Verification items for the finished model (mm, model axes). Coordinates: 2 decimals unless noted, no trailing zeros. Write each loop counter-clockwise with the first axis right and the second up, starting at its lowest first coordinate (ties: lowest second). Pieces come first, ordered by that corner, then holes. Notation, with made-up numbers: M 79.25,69 L 93.25,69 A21 cw 93.25,77 Z; hole C -30.75,19 d8. An arc over 180 degrees is marked long. Answer in a Markdown table with one row per item.
from build123d import *

# Parameters (mm, degrees)
SKETCH_1_R          = 20
EXTRUDE_1_DEPTH     = 20
SKETCH_4_R          = 2.5
CUT_EXTRUDE_1_DEPTH = 35.641016325
CHAMFER_1_SIZE      = 2
CHAMFER_1_SIZE2     = 1.154700538


with BuildPart() as part:
    # 草图1 → 凸台-拉伸1 (new body)
    with BuildSketch(Plane(origin=(0, 0, 0), x_dir=(1, 0, 0), z_dir=(0, 1, 0))):
        with Locations(Location((0, 0, 0), (0, 0, 270))):
            Circle(SKETCH_1_R)
    extrude(amount=EXTRUDE_1_DEPTH)

    # 草图2 → 切除-旋转1 (revolve, cut)
    with BuildSketch(Plane(origin=(0, 20, 0), x_dir=(1, 0, 0), z_dir=(0, 1, 0))):
        with BuildLine():
            Line((0, -3), (0, -23))
            ThreePointArc((0, -23), (-10, -13), (0, -3))
        make_face()
    revolve(axis=Axis((0, 20, 3), (0, 0, 1)), mode=Mode.SUBTRACT)

    # 草图4 → 切除-拉伸1 (cut, through all)
    with BuildSketch(Plane.XZ):
        with Locations(Location((0, -11.5, 0), (0, 0, 270))):
            Circle(SKETCH_4_R)
        with Locations(Location((11.5, 0, 0), (0, 0, 270))):
            Circle(SKETCH_4_R)
        with Locations(Location((-11.5, 0, 0), (0, 0, 270))):
            Circle(SKETCH_4_R)
    extrude(amount=-CUT_EXTRUDE_1_DEPTH, mode=Mode.SUBTRACT)

    # 倒角1
    chamfer_1_edges = [part.edges().sort_by_distance(p)[0] for p in [
        (0, 0, -9),
        (11.5, 0, 2.5),
        (-11.5, 0, 2.5),
    ]]
    chamfer_1_side = [part.faces().sort_by_distance(p)[0] for p in [
        (0, 0, 0.18852459),
    ]]
    chamfer(chamfer_1_edges, length=CHAMFER_1_SIZE, length2=CHAMFER_1_SIZE2, reference=chamfer_1_side[0])


solid = part.part
1) Thickness scan on L1, parallel to X at y = 13, z = 0; L2, parallel to X at y = 11.25, z = -0.5; L3, parallel to Z at x = 2, y = 11.5. Record the ranges inside material, lowest first. Write a range as [from, to].
Response values:
| item | result |
|---|---|
| L1 | x = [-20, -14], [-9, 9], [14, 20] |
| L2 | x = [-19.99, -13.95], [-9.05, 9.05], [13.95, 19.99] |
| L3 | z = [-19.9, -13], [-10, 8.13], [17.87, 19.9] |
2) Depth check by flat-ended pin: pin 1 (1.5 mm diameter, centred on x = 13.5, z = -2.5, fed in from -Y); pin 2 (3 mm diameter, centred on x = 11, y = 13.5, fed in from +Z); pin 3 (6 mm diameter, centred on y = 7.5, z = -11, fed in from +X); pin 4 (12 mm diameter, centred on x = 5, y = 7.5, fed in from -Z). Enter the tip coordinate at first touch or a pass-through.
Response values:
| item | result |
|---|---|
| pin 1 | stops at y = 0.32 |
| pin 2 | stops at z = 17.6 |
| pin 3 | stops at x = 18.33 |
| pin 4 | stops at z = -20 |
3) Release check for a two-part mould opening along Z. For faces 1 (the face through (0, 10, -9)), 2 (the face through (-13.94, 10.45, 0.54)), 3 (the face through (0, 20, -5)), 4 (the face through (0.88, 9.86, -19.98)) record: +Z half, -Z half, draft (parallel to the pull), parting line (faces both ways), or undercut.
Response values:
| item | result |
|---|---|
| face 1 | undercut |
| face 2 | undercut |
| face 3 | draft |
| face 4 | parting line |
4) Sectioned sample at D-D (y = 15.25). Record the cut outline in (x, z), then the cut area to 3 significant figures.
Response values:
| item | result |
|---|---|
| outline | M -6.52,18.91 A20 ccw long 6.52,18.91 A8.8 cw long Z; hole C -11.5,0 d5; hole C 0,-11.5 d5; hole C 11.5,0 d5 |
| area | 971 mm² |
5) Sectioned sample at B-B (z = 0). Record the cut outline in (x, y), then the cut area to 3 significant figures.
Response values:
| item | result |
|---|---|
| outline | M -20,0 L -16,0 L -14,1.15 L -14,20 L -20,20 Z; M -9,1.15 L -7,0 L 7,0 L 9,1.15 L 9,20 L -9,20 Z; M 14,1.15 L 16,0 L 20,0 L 20,20 L 14,20 Z |
| area | 595 mm² |
6) Sectioned sample at C-C (z = -11.5). Record the cut outline in (x, y), then the cut area to 3 significant figures.
Response values:
| item | result |
|---|---|
| outline | M -16.36,0 L -4.5,0 L -2.5,1.15 L -2.5,20 L -16.36,20 Z; M 2.5,1.15 L 4.5,0 L 16.36,0 L 16.36,20 L 2.5,20 Z |
| area | 552 mm² |
7) Sectioned sample at A-A (x = 0). Record the cut outline in (y, z).
Response values:
| item | result |
|---|---|
| outline | M 0,-20 L 20,-20 L 20,-14 L 1.15,-14 L 0,-16 Z; M 0,-7 L 1.15,-9 L 20,-9 L 20,3 A10 cw 12.86,20 L 0,20 Z |
